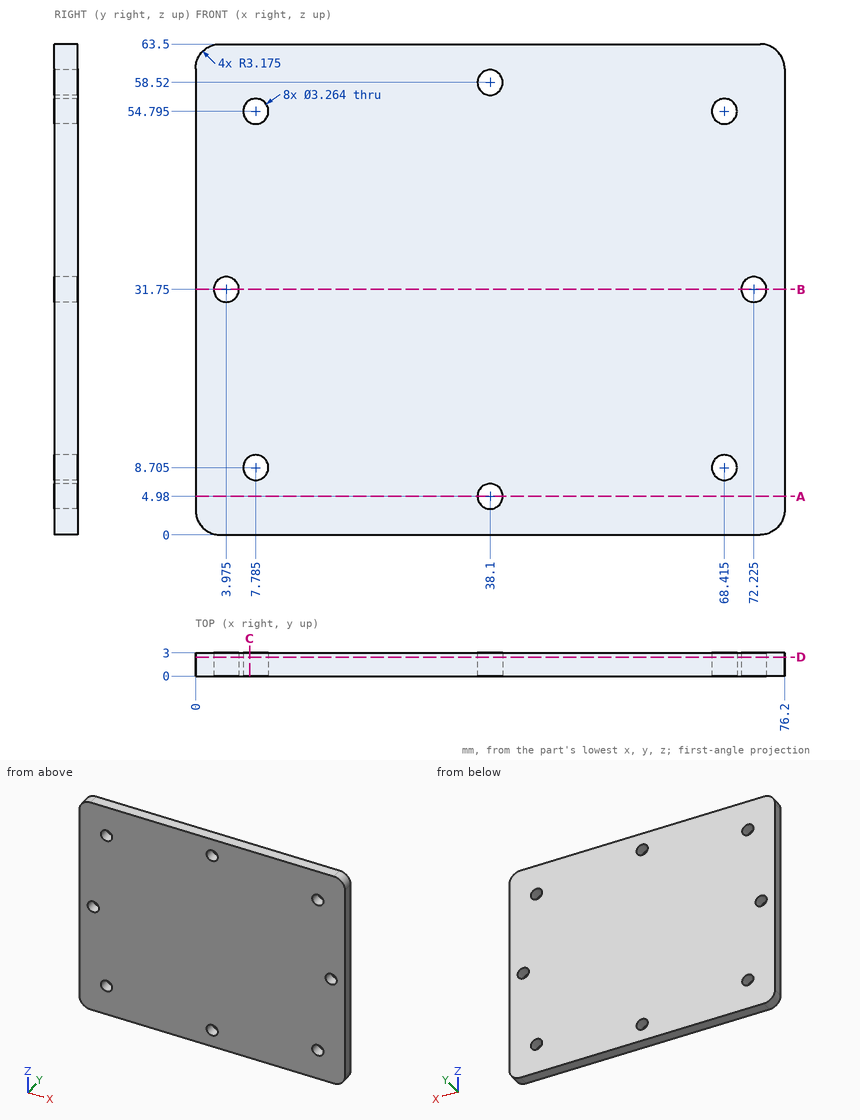
Verification items for this drawing (mm, ordinates from the low corner). Round coordinates to 2 decimals unless told otherwise and drop trailing zeros. Loops run counter-clockwise (first coordinate to the right, second up) from the corner with the lowest first, then second, coordinate; pieces in that order, holes last. Notation, with made-up numbers: M 8.25,7.25 L 66.25,7.25 A21 ccw 66.25,42.25 Z; hole C 14.25,-25 d1. An arc over 180 degrees is marked long. Answer as a JSON object with one key per item and string values.
1. Gauge pin test, flat end, axial feed: P1, Ø3, axis at x = 38.1, z = 58.52, coming from the -Y side. Record the tip position at first contact, or that the pin passes through.
Reply:
{"P1": "passes through"}
2. Section check C-C (x = 7). Record the boundary of the cut face in (y, z).
Reply:
{"outline": "M 0,0 L 3,0 L 3,7.27 L 0,7.27 Z; M 0,10.14 L 3,10.14 L 3,53.36 L 0,53.36 Z; M 0,56.23 L 3,56.23 L 3,63.5 L 0,63.5 Z"}
3. Section check B-B (z = 31.75). Record the boundary of the cut face in (x, y), plus the area to 3 significant figures.
Reply:
{"outline": "M 0,0 L 2.34,0 L 2.34,3 L 0,3 Z; M 5.61,0 L 70.59,0 L 70.59,3 L 5.61,3 Z; M 73.86,0 L 76.2,0 L 76.2,3 L 73.86,3 Z", "area": "209 mm²"}
4. Scan lines: line 1 (Z direction, x = 38.1, y = 0.95); line 2 (X direction, y = 0.6, z = 58.52); line 3 (X direction, y = 0.85, z = 3.5). Record each from-to range of solid material in increasing order.
Reply:
{"line 1": "z = 0 to 3.35, 6.61 to 56.89, 60.15 to 63.5", "line 2": "x = 0 to 36.47, 39.73 to 76.2", "line 3": "x = 0 to 37.41, 38.79 to 76.2"}
5. Section check A-A (z = 4.98). Record the boundary of the cut face in (x, y), plus the area to 3 significant figures.
Reply:
{"outline": "M 0,0 L 36.47,0 L 36.47,3 L 0,3 Z; M 39.73,0 L 76.2,0 L 76.2,3 L 39.73,3 Z", "area": "219 mm²"}
6. Section check D-D (y = 2.45). State how many separate pieces and enclosed holes the cut face has, plus the area to 3 significant figures.
Reply:
{"separate pieces": "1", "enclosed holes": "8", "area": "4,760 mm²"}
